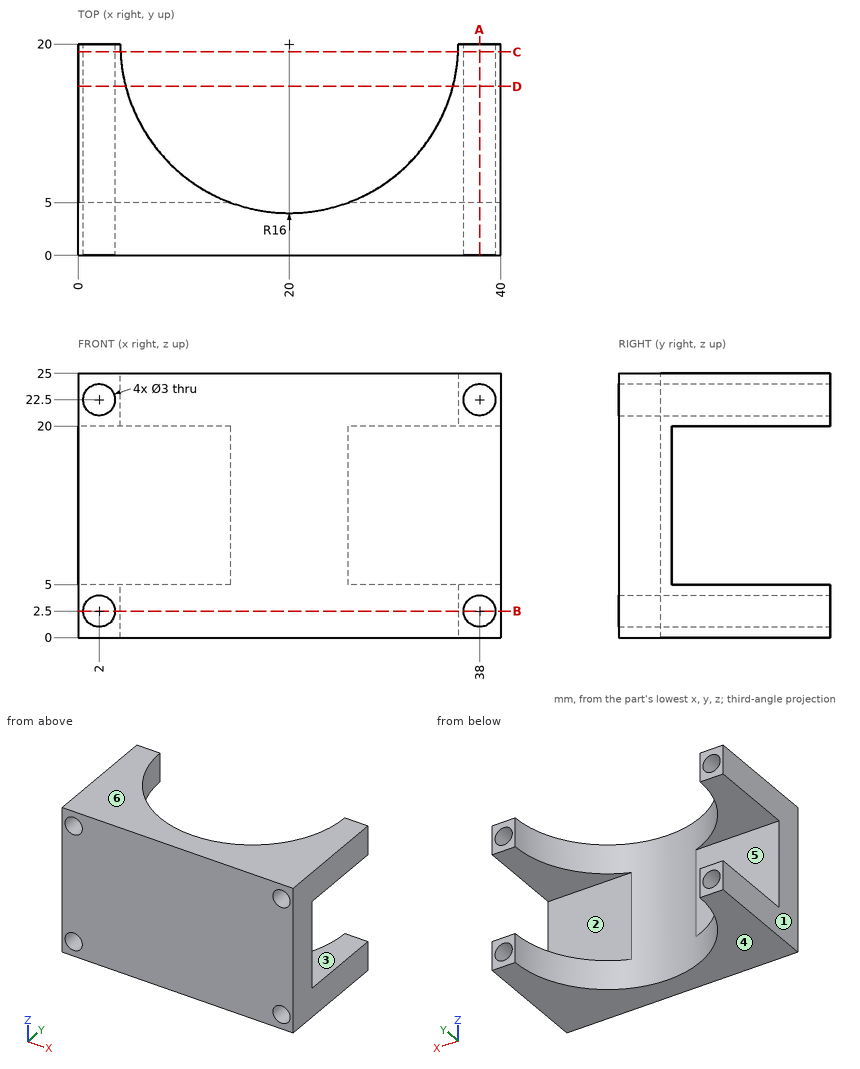
Here's the drawing with two shaded views (mm, measured from the low corner). I have some questions. A direction names the side the tool comes from. Give positions to 0.01 mm unless a question says otherwise; leave off trailing zeros. Loops run counter-clockwise (first coordinate to the right, second up) from the corner with the lowest first, then second, coordinate; pieces in that order, holes last. Notation, with made-up numbers: M 29.25,42 L 37.25,42 A28 cw 37.25,80 Z; hole C 19,-10 d8. An arc over 180 degrees is marked long. Use one line per item in the form item = value. Start each with the question number.
Q1. If we section it at D-D (y = 16): Write out the boundary of the cut face in (x, z), then the cut area to 3 significant figures.
Q2. I need wall thicknesses on line 1 along Z through (x, y) = (2, 10); line 2 along X through (y, z) = (9.75, 22.5); line 3 along X through (y, z) = (8.5, 3.75). Which ranges of each line are inside material? Lowest first, please.
Q3. If we section it at C-C (y = 19.25): Write out the boundary of the cut face in (x, z), then the cut area to 3 significant figures.
Q4. If we section it at A-A (x = 38): Write out the boundary of the cut face in (y, z).
Q5. Will these pins go through, and if not, where does the flat tip stop? pin 1 Ø1 at (x, z) = (6, 18) entering from +Y; pin 2 Ø6 at (x, z) = (14.5, 6.5) entering from +Y.
Q6. Thinking about a two-plate mould opening in Z: for the marked faces 1, 2, 3 and 4, which applies, +Z half, -Z half, draft (parallel to the pull), parting line (faces both ways), or undercut?
Q7. Which directions (+Z, -Z, +X, -X, +Y, -Y) give clear straight access to the entire face, cutting with the end or side of a thin tool? Please do the marked faces 5 and 6.
Q8. If we section it at B-B (z = 2.5): Write out the boundary of the cut face in (x, y).
Taken from the geometry:
q1.outline = M 0,0 L 4.51,0 L 4.51,5 L 0,5 Z; M 0,20 L 4.51,20 L 4.51,25 L 0,25 Z; M 35.49,0 L 40,0 L 40,5 L 35.49,5 Z; M 35.49,20 L 40,20 L 40,25 L 35.49,25 Z; hole C 2,2.5 d3; hole C 2,22.5 d3; hole C 38,2.5 d3; hole C 38,22.5 d3
q1.area = 61.9 mm^2
q2.line_1 = 0 to 1, 4 to 5, 20 to 21, 24 to 25
q2.line_2 = 0 to 0.5, 3.5 to 7.71, 32.29 to 36.5, 39.5 to 40
q2.line_3 = 0 to 1.17, 2.83 to 8.88, 31.12 to 37.17, 38.83 to 40
q3.outline = M 0,0 L 4.02,0 L 4.02,5 L 0,5 Z; M 0,20 L 4.02,20 L 4.02,25 L 0,25 Z; M 35.98,0 L 40,0 L 40,5 L 35.98,5 Z; M 35.98,20 L 40,20 L 40,25 L 35.98,25 Z; hole C 2,2.5 d3; hole C 2,22.5 d3; hole C 38,2.5 d3; hole C 38,22.5 d3
q3.area = 52.1 mm^2
q4.outline = M 0,0 L 20,0 L 20,1 L 0,1 Z; M 0,4 L 20,4 L 20,5 L 5,5 L 5,20 L 20,20 L 20,21 L 0,21 Z; M 0,24 L 20,24 L 20,25 L 0,25 Z
q5.pin_1 = 5
q5.pin_2 = 6.2
q6.face_1 = draft
q6.face_2 = undercut
q6.face_3 = undercut
q6.face_4 = -Z half
q7.face_5 = +X, -X, +Y
q7.face_6 = +Z, +X, -X, +Y, -Y
q8.outline = M 0,0 L 0.5,0 L 0.5,20 L 0,20 Z; M 3.5,0 L 36.5,0 L 36.5,20 L 36,20 A16 cw 4,20 L 3.5,20 Z; M 39.5,0 L 40,0 L 40,20 L 39.5,20 Z
